Drawing for the job (mm, zero at the part's lowest x, y, z). Round coordinates to 2 decimals unless told otherwise and drop trailing zeros. Order: outer loops, then holes, each group sorted by start corner. A loop starts at its lowest first (then second) coordinate and runs counter-clockwise, first axis right, second up. Notation, with made-up numbers: (-18, 4.5) - (14, 4.5) arc R13 ccw to (14, 17.5) - close; hole circle Ø9 at (53.25, -21). An arc over 180 degrees is marked (long way). Answer as a JSON object with one key per item and string values.
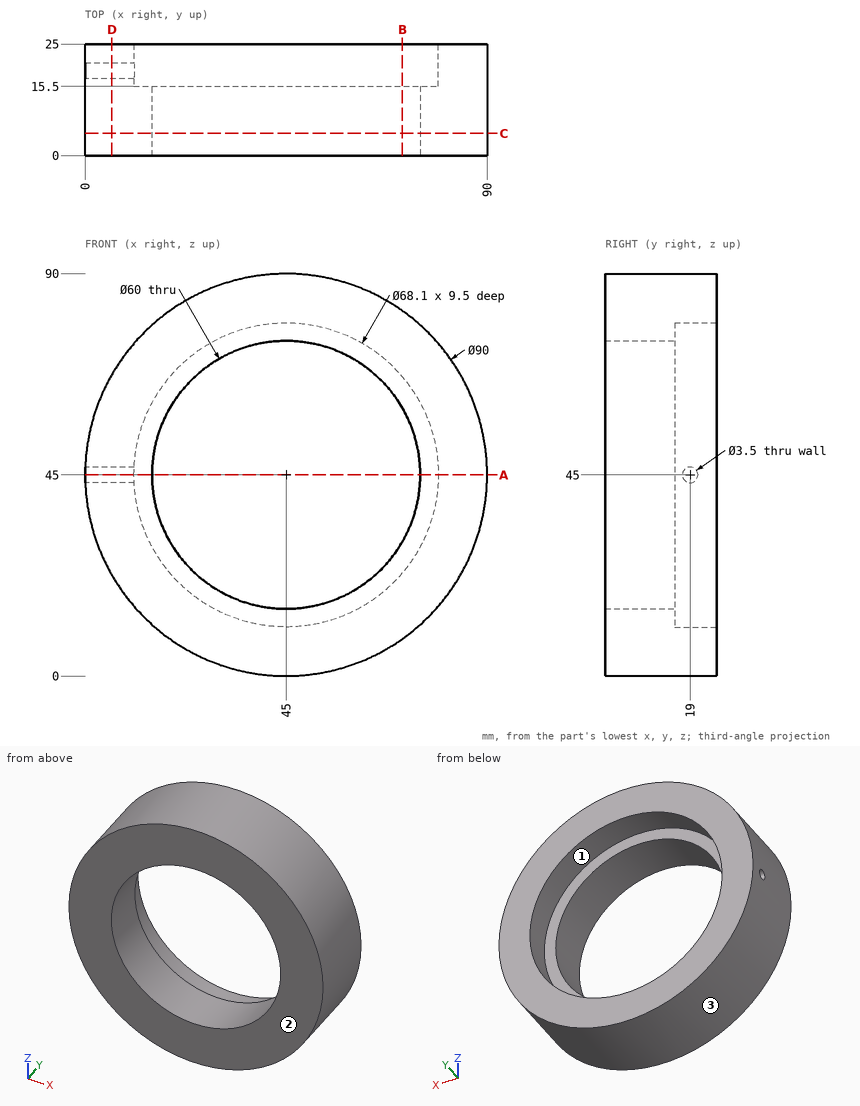
Item 1: Cut at C-C (y = 5). Write the cut outline in (x, z), plus the area to 3 significant figures.
Taken from the geometry:
{"outline": "circle Ø90 at (45, 45); hole circle Ø60 at (45, 45)", "area": "3,530 mm2"}
Item 2: Probe L1, parallel to Z at x = 45, y = 9; L2, parallel to Z at x = 45, y = 20.75; L3, parallel to X at y = 20.5, z = 34.5. List the from-to ranges inside material, lowest first. Write a range as from..to.
Taken from the geometry:
{"L1": "0..15, 75..90", "L2": "0..10.95, 79.05..90", "L3": "1.24..12.61, 77.39..88.76"}
Item 3: Cut at B-B (x = 71). Write the cut outline in (y, z).
Taken from the geometry:
{"outline": "(0, 8.27) - (25, 8.27) - (25, 23.01) - (15.5, 23.01) - (15.5, 30.03) - (0, 30.03) - close; (0, 59.97) - (15.5, 59.97) - (15.5, 66.99) - (25, 66.99) - (25, 81.73) - (0, 81.73) - close"}
Item 4: Two-plate mould, pull along Z, no slides. Class the marked faces 1, 2 and 3: pulls with the +Z half, pulls with the -Z half, needs draft (parallel to the pull), parting line crosses it, or undercut.
Taken from the geometry:
{"face 1": "undercut", "face 2": "needs draft", "face 3": "parting line crosses it"}
Item 5: Cut at A-A (z = 45). Write the cut outline in (x, y).
Taken from the geometry:
{"outline": "(0, 0) - (15, 0) - (15, 15.5) - (10.95, 15.5) - (10.95, 17.25) - (0, 17.25) - close; (0, 20.75) - (10.95, 20.75) - (10.95, 25) - (0, 25) - close; (75, 0) - (90, 0) - (90, 25) - (79.05, 25) - (79.05, 15.5) - (75, 15.5) - close"}
Item 6: Drop flat-ended pins along their axis: P1, Ø5, axis at x = 54.5, y = 8, coming from the +Z side; P2, Ø12, axis at y = 8.5, z = 32.5, coming from the -X side; P3, Ø5, axis at x = 52.5, z = 16.5, coming from the -Y side; P4, Ø1, axis at x = 21, y = 16.5, coming from the +Z side. Give the stop position or say it passes through.
Taken from the geometry:
{"P1": "z = 89.45", "P2": "x = 0.47", "P3": "y = 0", "P4": "z = 83.38"}
Item 7: Cut at D-D (x = 6). Write the cut outline in (y, z).
Taken from the geometry:
{"outline": "(0, 22.55) - (25, 22.55) - (25, 67.45) - (0, 67.45) - close; hole circle Ø3.5 at (19, 45)"}
